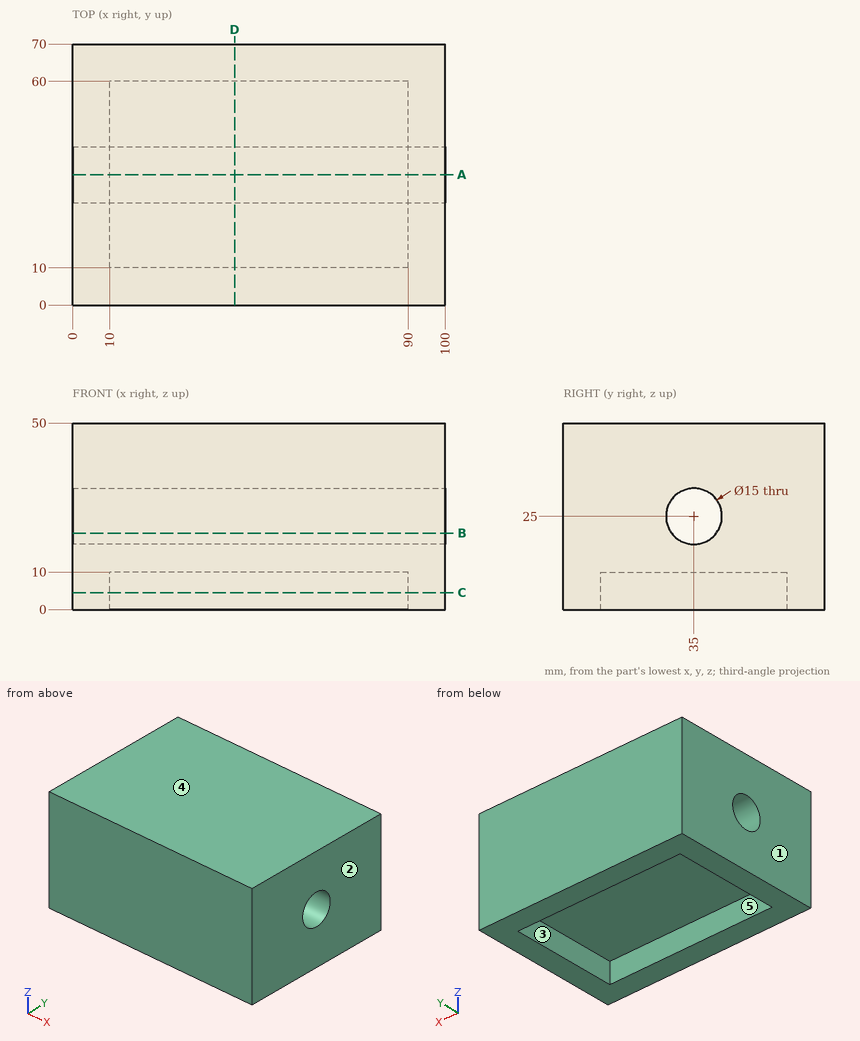
Input: dimensioned drawing with shaded views. Units: mm. Origin: part minimum x, y, z. A direction names the side the tool comes from. Round coordinates to 2 decimals unless told otherwise and drop trailing zeros. Order: outer loops, then holes, each group sorted by start corner. A loop starts at its lowest first (then second) coordinate and runs counter-clockwise, first axis right, second up.
1. Pin query (flat end, axial travel): P1, Ø1.5, axis at x = 58.5, z = 44.5, coming from the -Y side; P2, Ø2, axis at x = 44.5, y = 32, coming from the -Z side. Return the tip coordinate at first contact, or that it passes through.
The answers:
P1: stops at y = 0
P2: stops at z = 10
2. Cut plane B-B, the plane z = 20.5. Output: boundary loops of the cut face in (x, y).
The answers:
outline: (0, 0) - (100, 0) - (100, 29) - (0, 29) - close; (0, 41) - (100, 41) - (100, 70) - (0, 70) - close
3. Material intervals for line 1 (Y direction, x = 46, z = 25); line 2 (Y direction, x = 16, z = 7); line 3 (Z direction, x = 85.5, y = 35.5), sorted ascending.
The answers:
line 1: y = 0 to 27.5, 42.5 to 70
line 2: y = 0 to 10, 60 to 70
line 3: z = 10 to 17.52, 32.48 to 50
4. Cut plane C-C, the plane z = 4.5. Output: boundary loops of the cut face in (x, y), then the cut area to 3 significant figures.
The answers:
outline: (0, 0) - (100, 0) - (100, 70) - (0, 70) - close; hole (10, 10) - (90, 10) - (90, 60) - (10, 60) - close
area: 3,000 mm2
5. Mould query, pull axis X, two halves, no side actions, for the marked faces 1, 2 and 3. Classes: released by +X, released by -X, zero draft, split by the parting line, or undercut.
The answers:
face 1: released by -X
face 2: released by +X
face 3: undercut
6. Set-up query: the marked faces 4 and 5. Return all of +Z, -Z, +X, -X, +Y, -Y with unobstructed straight access to the full face (end or side cutting, diameter ignored); none if empty.
The answers:
face 4: +Z, +X, -X, +Y, -Y
face 5: -Z
7. Cut plane D-D, the plane x = 43.5. Output: boundary loops of the cut face in (y, z), then the cut area to 3 significant figures.
The answers:
outline: (0, 0) - (10, 0) - (10, 10) - (60, 10) - (60, 0) - (70, 0) - (70, 50) - (0, 50) - close; hole circle Ø15 at (35, 25)
area: 2,820 mm2
8. Cut plane A-A, the plane y = 35. Output: boundary loops of the cut face in (x, z).
The answers:
outline: (0, 0) - (10, 0) - (10, 10) - (90, 10) - (90, 0) - (100, 0) - (100, 17.5) - (0, 17.5) - close; (0, 32.5) - (100, 32.5) - (100, 50) - (0, 50) - close
